Work out the finished part from the listing and answer in its coordinate system (mm). Face numbers are marked on the shaded views. A direction names the side the tool comes from. Round coordinates to 2 decimals unless told otherwise and drop trailing zeros. Write each loop counter-clockwise with the first axis right and the second up, starting at its lowest first coordinate (ties: lowest second). Pieces come first, ordered by that corner, then holes. Notation, with made-up numbers: (-18, 15.5) - (28, 15.5) arc R21 cw to (28, 42.5) - close; hole circle Ø7 at (-8, 31.5). An arc over 180 degrees is marked (long way). Answer as a JSON object with one key per item and string values.
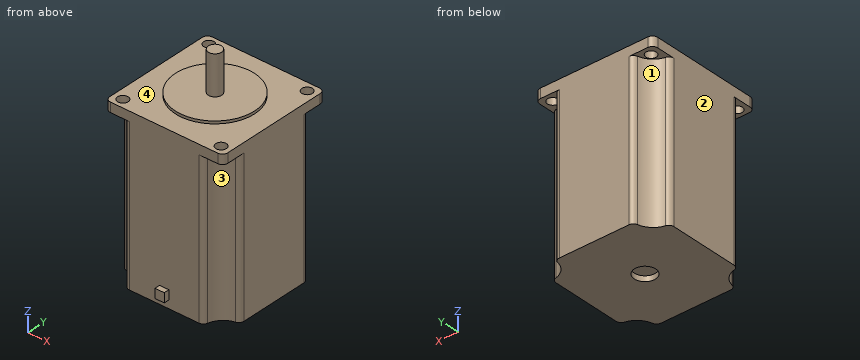
```python
from build123d import *

# Parameters (mm, degrees)
BOSS_EXTRUDE1_DEPTH = 4.572
SKETCH2_R           = 2.5
SKETCH2_R_2         = 2.54
CUT_EXTRUDE1_DEPTH  = 12.7
SKETCH3_R           = 3.175
BOSS_EXTRUDE2_DEPTH = 20
BOSS_EXTRUDE3_DEPTH = 73.152
SKETCH7_R           = 5.08
CUT_EXTRUDE2_DEPTH  = 2.54
SKETCH8_W           = 4.445
SKETCH8_H           = 4.445
BOSS_EXTRUDE4_DEPTH = 2.54
SKETCH9_R           = 18.923
BOSS_EXTRUDE5_DEPTH = 1.27


with BuildPart() as part:
    # Sketch1 → Boss-Extrude1 (new body)
    with BuildSketch(Plane.XY):
        with BuildLine():
            Line((-25.66, 28.194), (25.66, 28.194))
            ThreePointArc((25.66, 28.194), (27.456051224, 27.450051224), (28.2, 25.654))
            Line((28.2, 25.654), (28.2, -25.654))
            ThreePointArc((28.2, -25.654), (27.456051224, -27.450051224), (25.66, -28.194))
            Line((25.66, -28.194), (-25.66, -28.194))
            ThreePointArc((-25.66, -28.194), (-27.456051224, -27.450051224), (-28.2, -25.654))
            Line((-28.2, -25.654), (-28.2, 25.654))
            ThreePointArc((-28.2, 25.654), (-27.456051224, 27.450051224), (-25.66, 28.194))
        make_face()
    extrude(amount=-BOSS_EXTRUDE1_DEPTH)

    # Sketch2 → Cut-Extrude1 (cut)
    with BuildSketch(Plane.XY):
        with Locations((-23.495, 23.876)):
            Circle(SKETCH2_R)
        with Locations((23.505, 23.876)):
            Circle(SKETCH2_R_2)
        with Locations((-23.495, -23.876)):
            Circle(SKETCH2_R_2)
        with Locations((23.505, -23.876)):
            Circle(SKETCH2_R_2)
    extrude(amount=-CUT_EXTRUDE1_DEPTH, mode=Mode.SUBTRACT)

    # Sketch3 → Boss-Extrude2 (add)
    with BuildSketch(Plane.XY):
        Circle(SKETCH3_R)
    extrude(amount=BOSS_EXTRUDE2_DEPTH)

    # Sketch6 → Boss-Extrude3 (add)
    with BuildSketch(Plane(origin=(0, 0, -4.572), x_dir=(-1, 0, 0), z_dir=(0, 0, -1))):
        with BuildLine():
            Line((-16.59544611, 28.194), (16.59544611, 28.194))
            ThreePointArc((16.59544611, 28.194), (18.187513991, 27.633120982), (19.076465755, 26.198188868))
            ThreePointArc((19.076465755, 26.198188868), (21.596845623, 21.593151837), (26.203044563, 19.07489608))
            ThreePointArc((26.203044563, 19.07489608), (27.638753799, 18.186149944), (28.2, 16.59362572))
            Line((28.2, 16.59362572), (28.2, -16.59362572))
            ThreePointArc((28.2, -16.59362572), (27.638442141, -18.186537109), (26.202073469, -19.075108412))
            ThreePointArc((26.202073469, -19.075108412), (21.595673614, -21.592228782), (19.076199379, -26.19734161))
            ThreePointArc((19.076199379, -26.19734161), (18.187399824, -27.632849121), (16.594994048, -28.194))
            Line((16.594994048, -28.194), (-16.594994048, -28.194))
            ThreePointArc((-16.594994048, -28.194), (-18.18696432, -27.633199499), (-19.075960003, -26.198433587))
            ThreePointArc((-19.075960003, -26.198433587), (-21.596706334, -21.593572144), (-26.203011658, -19.07546527))
            ThreePointArc((-26.203011658, -19.07546527), (-27.638743239, -18.186725052), (-28.2, -16.594187708))
            Line((-28.2, -16.594187708), (-28.2, 16.594187708))
            ThreePointArc((-28.2, 16.594187708), (-27.638751536, 18.186714743), (-26.203037512, 19.075459612))
            ThreePointArc((-26.203037512, 19.075459612), (-21.596941467, 21.593557838), (-19.076433541, 26.198335711))
            ThreePointArc((-19.076433541, 26.198335711), (-18.187455421, 27.633168096), (-16.59544611, 28.194))
        make_face()
    extrude(amount=BOSS_EXTRUDE3_DEPTH)

    # Sketch7 → Cut-Extrude2 (cut)
    with BuildSketch(Plane(origin=(0, 0, -77.724), x_dir=(-1, 0, 0), z_dir=(0, 0, -1))):
        Circle(SKETCH7_R)
    extrude(amount=-CUT_EXTRUDE2_DEPTH, mode=Mode.SUBTRACT)

    # Sketch8 → Boss-Extrude4 (add)
    with BuildSketch(Plane(origin=(0, -28.194, 0), x_dir=(-1, 0, 0), z_dir=(0, -1, 0))):
        with Locations((0, 71.6915)):
            Rectangle(SKETCH8_W, SKETCH8_H)
    extrude(amount=BOSS_EXTRUDE4_DEPTH)

    # Sketch9 → Boss-Extrude5 (add)
    with BuildSketch(Plane.XY):
        Circle(SKETCH9_R)
    extrude(amount=BOSS_EXTRUDE5_DEPTH)


solid = part.part
```
Item 1: A cutting plane is placed at C-C (x = 0). Write down the section's boundary in (y, z) (3 decimals), and give its area (3 significant figures).
Results found:
{"outline": "(-30.734, -73.914) - (-28.194, -73.914) - (-28.194, -77.724) - (-5.08, -77.724) - (-5.08, -75.184) - (5.08, -75.184) - (5.08, -77.724) - (28.194, -77.724) - (28.194, 0) - (18.923, 0) - (18.923, 1.27) - (3.175, 1.27) - (3.175, 20) - (-3.175, 20) - (-3.175, 1.27) - (-18.923, 1.27) - (-18.923, 0) - (-28.194, 0) - (-28.194, -69.469) - (-30.734, -69.469) - close", "area": "4,540 mm²"}
Item 2: A cutting plane is placed at B-B (y = 0). Write down the section's boundary in (x, z) (3 decimals).
Results found:
{"outline": "(-28.2, -77.724) - (-5.08, -77.724) - (-5.08, -75.184) - (5.08, -75.184) - (5.08, -77.724) - (28.2, -77.724) - (28.2, 0) - (18.923, 0) - (18.923, 1.27) - (3.175, 1.27) - (3.175, 20) - (-3.175, 20) - (-3.175, 1.27) - (-18.923, 1.27) - (-18.923, 0) - (-28.2, 0) - close"}
Item 3: Each of these flat-tipped pins is pushed along its axis until it touches: P1, Ø6, axis at x = -23.495, y = 23.876, coming from the +Z side; P2, Ø19, axis at x = 5, y = 6, coming from the +Z side; P3, Ø1.3, axis at x = -0.5, y = -30, coming from the -Z side; P4, Ø3, axis at y = -29, z = -72, coming from the +X side. Where does it stop, or does it pass through?
Results found:
{"P1": "z = 0", "P2": "z = 20", "P3": "z = -73.91", "P4": "x = 18.34"}
Item 4: A cutting plane is placed at A-A (z = -41). Write down the section's boundary in (x, y) (3 decimals), and give its area (3 significant figures).
Results found:
{"outline": "(-28.2, -16.594) arc R2.54 ccw to (-26.202, -19.075) arc R9.334 cw to (-19.076, -26.197) arc R2.54 ccw to (-16.595, -28.194) - (16.595, -28.194) arc R2.54 ccw to (19.076, -26.198) arc R9.341 cw to (26.203, -19.075) arc R2.54 ccw to (28.2, -16.594) - (28.2, 16.594) arc R2.54 ccw to (26.203, 19.075) arc R9.341 cw to (19.076, 26.198) arc R2.54 ccw to (16.595, 28.194) - (-16.595, 28.194) arc R2.54 ccw to (-19.076, 26.198) arc R9.34 cw to (-26.203, 19.075) arc R2.54 ccw to (-28.2, 16.594) - close", "area": "2,900 mm²"}
Item 5: Consider line 1 along Y through (x, z) = (-0.5, -53.5); line 2 along Z through (x, y) = (20, 21.5); line 3 along Z through (x, y) = (26.5, -26). Determine where each line is inside the solid, lowest interval first.
Results found:
{"line 1": "-28.19 to 28.19", "line 2": "-77.72 to 0", "line 3": "-4.57 to 0"}
Item 6: A cutting plane is placed at D-D (y = -15). Write down the section's boundary in (x, z), and give its area (3 significant figures).
Results found:
{"outline": "(-28.2, -77.72) - (28.2, -77.72) - (28.2, 0) - (11.54, 0) - (11.54, 1.27) - (-11.54, 1.27) - (-11.54, 0) - (-28.2, 0) - close", "area": "4,410 mm²"}
Item 7: For the marked faces 1, 2, 3 and 4, determine the directions among +Z, -Z, +X, -X, +Y, -Y from which every point of the face is accessible in a straight line to the end or side of a thin tool.
Results found:
{"face 1": "-Z, -X, +Y", "face 2": "+Z, -Z, -X, +Y, -Y", "face 3": "-Z, +X, -Y", "face 4": "+Z"}
